Could you check a few things on this model? Use its own coordinates, in mm. A direction names the side the tool comes from. Coordinates: 2 decimals unless noted, no trailing zeros. Write each loop counter-clockwise with the first axis right and the second up, starting at its lowest first coordinate (ties: lowest second). Pieces come first, ordered by that corner, then holes.
```python
from build123d import *

# Parameters (mm, degrees)
F0_W      = 35
F0_H      = 70
F1_DEPTH  = 40
F2_W      = 20.5
F2_H      = 55.6
F3_DEPTH  = 35
F4_W      = 20.5
F4_H      = 40.5
F5_DEPTH  = 25
F6_DEPTH  = 6
F7_W      = 3.5
F7_H      = 6
F8_DEPTH  = 3.5
F10_D     = 4.2
F10_DEPTH = 15
F10_TIP   = 1.2618073
F11_R     = 2
F12_W     = 9
F12_H     = 6
F13_DEPTH = 10


# Not quite as in the source:
# - a pattern or mirror of a feature is missing from the dataset's text; its kind, count and spacing are read off the source's solid


with BuildPart() as f1:
    # F0 (on Top) → F1 (new body)
    with BuildSketch(Plane.XY):
        Rectangle(F0_W, F0_H)
    extrude(amount=F1_DEPTH)

    # F2 (on face) → F3 (cut)
    with BuildSketch(Plane(origin=(0, 0, 0), x_dir=(1, 0, 0), z_dir=(0, 0, -1))):
        Rectangle(F2_W, F2_H)
    extrude(amount=-F3_DEPTH, mode=Mode.SUBTRACT)

    # F4 (on face) → F5 (cut)
    with BuildSketch(Plane.XY.offset(40)):
        Rectangle(F4_W, F4_H)
    extrude(amount=-F5_DEPTH, mode=Mode.SUBTRACT)

    # F6 (cut): a face of the model
    f6_faces = [f1.faces().sort_by_distance(p)[0] for p in [
        (16.7173762079, 0, 0),
    ]]
    extrude(f6_faces, amount=-F6_DEPTH, mode=Mode.SUBTRACT)

    # F7 (on face) → F8 (cut)
    with BuildSketch(Plane(origin=(0, 0, 35), x_dir=(1, 0, 0), z_dir=(0, 0, -1))):
        with Locations((0, 23.25)):
            Rectangle(F7_W, F7_H)
    f8 = extrude(amount=-F8_DEPTH, mode=Mode.SUBTRACT)

    # F8_copies: F8 across plane
    add(f8.mirror(Plane.ZX), mode=Mode.SUBTRACT)

    # F10
    with Locations(Plane(origin=(0, 0, 6), x_dir=(1, 0, 0), z_dir=(0, 0, -1))):
        with Locations((-13.875, 31.4), (13.875, 31.4), (13.875, -31.4), (-13.875, -31.4)):
            Hole(F10_D / 2, depth=F10_DEPTH)
            with Locations((0, 0, -(F10_DEPTH + F10_TIP / 2))):  # 118° drill point
                Cone(0, F10_D / 2, F10_TIP, mode=Mode.SUBTRACT)

    # F11
    f11_edges = [f1.edges().sort_by_distance(p)[0] for p in [
        (17.5, -35, 23),
        (17.5, 0, 40),
        (0, -35, 40),
        (-17.5, 0, 40),
        (17.5, 35, 23),
        (0, 35, 40),
        (-17.5, -35, 23),
        (-17.5, 35, 23),
    ]]
    fillet(f11_edges, radius=F11_R)

    # F12 (on face) → F13 (cut)
    with BuildSketch(Plane(origin=(0, 35, 0), x_dir=(-1, 0, 0), z_dir=(0, 1, 0))):
        with Locations((0, 9)):
            Rectangle(F12_W, F12_H)
    extrude(amount=-F13_DEPTH, mode=Mode.SUBTRACT)


solid = f1.part
```
Item 1: I want a section at C-C, the plane z = 11. List the corners of the cut face in (x, y) for me (3 decimals).
Item 2: If we mould it in two halves opening along X, with no side actions, what happens to faces 1 (the flat face through (-11, 0, 40)), 2 (the cylindrical face through (-16.93, 0.46, 39.4)), 3 (the cylindrical face through (-13.6, -33.48, 13.6))? For each: released by +X, released by -X, zero draft, split by the parting line, or undercut.
Item 3: Will these pins go through, and if not, where does the flat tip stop? pin 1 Ø3.5 at (x, y) = (-13.875, 31.4) entering from -Z; pin 2 Ø5 at (x, y) = (6.5, 22.5) entering from -Z; pin 3 Ø2 at (x, z) = (-1, 10.5) entering from +Y.
Item 4: If I drill on line 1 along Y through (x, z) = (-0.5, 15.5); line 2 along X through (y, z) = (-31.4, 15) (3 decimals); line 3 along X through (y, z) = (31, 17), over which ranges is the centre line in solid material (lowest first)?
Item 5: Which directions (+Z, -Z, +X, -X, +Y, -Y) give clear straight access to the entire face, cutting with the end or side of a thin tool? Please do faces 4 (the flat face through (4.5, 31, 9)), 5 (the flat face through (10.25, 0, 23)), 6 (the cylindrical face through (-16.93, 34.4, 22.22)).
Item 6: I want a section at A-A, the plane x = -0.5. List the corners of the cut face in (y, z) for me, then the cut area to 3 significant figures.
Item 7: I want a section at B-B, the plane y = -11. List the corners of the cut face in (x, z) for me, then the cut area to 3 significant figures.
Item 8: I want a section at D-D, the plane z = 28. List the corners of the cut face in (x, y) for me, then the cut area to 3 significant figures.
Taken from the geometry:
1. outline: (-17.5, -33) arc R2 ccw to (-15.5, -35) - (15.5, -35) arc R2 ccw to (17.5, -33) - (17.5, 33) arc R2 ccw to (15.5, 35) - (4.5, 35) - (4.5, 27.8) - (10.25, 27.8) - (10.25, -27.8) - (-10.25, -27.8) - (-10.25, 27.8) - (-4.5, 27.8) - (-4.5, 35) - (-15.5, 35) arc R2 ccw to (-17.5, 33) - close; hole circle Ø4.2 at (-13.875, -31.4); hole circle Ø4.2 at (-13.875, 31.4); hole circle Ø4.2 at (13.875, -31.4); hole circle Ø4.2 at (13.875, 31.4)
2. face 1: zero draft
2. face 2: released by -X
2. face 3: undercut
3. pin 1: stops at z = 21.21
3. pin 2: stops at z = 35
3. pin 3: stops at y = -27.8
4. line 1: y = -35 to -27.8, 27.8 to 35
4. line 2: x = -17.5 to -15.975, -11.775 to 11.775, 15.975 to 17.5
4. line 3: x = -17.5 to -15.94, -11.81 to 11.81, 15.94 to 17.5
5. face 4: -Z, +Y
5. face 5: -Z
5. face 6: +Z, -Z, -X, +Y
6. outline: (-35, 6) - (-27.8, 6) - (-27.8, 35) - (-26.25, 35) - (-26.25, 38.5) - (-20.25, 38.5) - (-20.25, 40) - (-33, 40) arc R2 ccw to (-35, 38) - close; (20.25, 38.5) - (26.25, 38.5) - (26.25, 35) - (27.8, 35) - (27.8, 12) - (35, 12) - (35, 38) arc R2 ccw to (33, 40) - (20.25, 40) - close
6. area: 478 mm2
7. outline: (-17.5, 6) - (-10.25, 6) - (-10.25, 40) - (-15.5, 40) arc R2 ccw to (-17.5, 38) - close; (10.25, 6) - (17.5, 6) - (17.5, 38) arc R2 ccw to (15.5, 40) - (10.25, 40) - close
7. area: 491 mm2
8. outline: (-17.5, -33) arc R2 ccw to (-15.5, -35) - (15.5, -35) arc R2 ccw to (17.5, -33) - (17.5, 33) arc R2 ccw to (15.5, 35) - (-15.5, 35) arc R2 ccw to (-17.5, 33) - close; hole (-10.25, -27.8) - (10.25, -27.8) - (10.25, 27.8) - (-10.25, 27.8) - close
8. area: 1,310 mm2
